Design review of the part built by this model. Coordinates are the model's own, in mm. A direction names the side the tool comes from. Round coordinates to 2 decimals unless told otherwise and drop trailing zeros. Loops run counter-clockwise (first coordinate to the right, second up) from the corner with the lowest first, then second, coordinate; pieces in that order, holes last. Notation, with made-up numbers: (-23, 33.5) - (-17, 33.5) arc R5 ccw to (-17, 41.5) - close; hole circle Ø6 at (28.5, 3). An arc over 180 degrees is marked (long way). Return JSON: item names as keys, results as strings. Group by question number.
(1) Wall thickness on L1, parallel to Z at x = 40, y = 46.75; L2, parallel to Y at x = -31, z = 3; L3, parallel to X at y = 126, z = 0.25: over which ranges is each line inside the solid? List them lowest first. Write a range as [from, to].
(2) We need section D-D, the plane x = 62.5. Write out the cut boundary in (y, z).
(3) We need section B-B, the plane x = -3. Write out the cut boundary in (y, z).
(4) Clearance check with flat-ended pins moving along their axes: pin 1 (4 mm diameter, centred on y = 27, z = -1.5, fed in from +X); pin 2 (6 mm diameter, centred on y = 47.5, z = 2, fed in from +X); pin 3 (10 mm diameter, centred on x = -44.5, y = 31.5, fed in from -Z); pin 4 (2.5 mm diameter, centred on y = 150.5, z = 0, fed in from +X). State where each tip first meets the part, or that it passes through.
(5) We need section C-C, the plane x = -27.5. Write out the cut boundary in (y, z).
(6) The part is to be moulded in two halves that separate along Y. For faces 1 (the flat face through (50, 20, 0)), 2 (the cylindrical face through (73.513, 30.085, 0.056)), 3 (the cylindrical face through (81.638, 112.718, -0.056)), say which applies: pulls with the +Y half, pulls with the -Y half, needs draft (parallel to the pull), parting line crosses it, or undercut.
(7) We need section A-A, the plane y = 85.5. Write out the cut boundary in (x, z), and give its area (3 significant figures).
(8) For faces 4 (the flat face through (1, 40, 0)), 5 (the cylindrical face through (65.185, 14.682, 0.596)), 6 (the flat face through (67.5, 10, 0)), 7 (the cylindrical face through (-0.66, 134.83, -0.06)), list the 3-axis set-ups (+Z, -Z, +X, -X, +Y, -Y) from which the entire face can be reached by the end or side of a thin tool; tool diameter is ignored.
Autodesk Inventor part; units mm, degrees
ref_plane "YZ Plane" through (0, 0, 0) normal (1, 0, 0) x (0, 1, 0)
ref_plane "XZ Plane" through (0, 0, 0) normal (0, 1, 0) x (-1, 0, 0)
ref_plane "XY Plane" through (0, 0, 0) normal (0, 0, 1) x (1, 0, 0)
sketch "Sketch2" plane through (0, 0, 0) normal (0, 0, 1) x (1, 0, 0)
  line L0 (-50, 0) -> (50, 0) construction
  line L1 (50, 0) -> (50, 40)
  line L2 (50, 40) -> (-50, 40)
  line L3 (-50, 40) -> (-50, 0)
  arc A0 (50, 0) -> (-50, 0) centre (0, 74.8331) ccw
  line L4 (57.5, 19.2117) -> (57.5, 34.9113)
  line L5 (-57.5, 34.9113) -> (-57.5, 19.2117)
  line L6 (7.5, 154.4808) -> (7.5, 144.4302)
  line L7 (-7.5, 154.4808) -> (-7.5, 144.4302)
  line L8 (7.5, 144.4302) -> (-7.5, 154.4808) construction
  arc A1 (57.5, 34.9113) -> (7.5, 144.4302) centre (0, 74.8331) ccw
  arc A2 (-7.5, 144.4302) -> (-57.5, 34.9113) centre (0, 74.8331) ccw
  arc A3 (57.5, 19.2117) -> (7.5, 154.4808) centre (0, 74.8331) ccw
  arc A4 (-7.5, 154.4808) -> (-57.5, 19.2117) centre (0, 74.8331) ccw
  line L9 (56.6273, 55) -> (45.8982, 55)
  line L10 (-45.8982, 55) -> (-56.6273, 55)
  line L11 (42.4264, 117.2596) -> (35.3553, 110.1885)
  line L12 (-35.3553, 110.1885) -> (-42.4264, 117.2596)
  line L13 (49.1491, 109.2477) -> (40.9576, 103.512)
  line L14 (-49.1491, 109.2477) -> (-40.9576, 103.512)
  arc A5 (-40.9576, 103.512) -> (-45.8982, 55) centre (0, 74.8331) ccw
  arc A6 (-49.1491, 109.2477) -> (-56.6273, 55) centre (0, 74.8331) ccw
  arc A7 (45.8982, 55) -> (40.9576, 103.512) centre (0, 74.8331) ccw
  arc A8 (35.3553, 110.1885) -> (-35.3553, 110.1885) centre (0, 74.8331) ccw
  arc A9 (56.6273, 55) -> (49.1491, 109.2477) centre (0, 74.8331) ccw
  arc A10 (42.4264, 117.2596) -> (-42.4264, 117.2596) centre (0, 74.8331) ccw
  line L15 (7.5, 114.1237) -> (7.5, 103.8805)
  line L16 (-7.5, 103.8805) -> (-7.5, 114.1237)
  line L17 (34.7368, 55) -> (22.5088, 55)
  line L18 (-22.5088, 55) -> (-34.7368, 55)
  arc A11 (-7.5, 103.8805) -> (-22.5088, 55) centre (0, 74.8331) ccw
  arc A12 (22.5088, 55) -> (7.5, 103.8805) centre (0, 74.8331) ccw
  arc A13 (-7.5, 114.1237) -> (-34.7368, 55) centre (0, 74.8331) ccw
  arc A14 (34.7368, 55) -> (7.5, 114.1237) centre (0, 74.8331) ccw
  point P0 (0, 0)
  point P1 (0, 0)
  point P2 (0, 149.4555)
  dimension "d11" = 100
  dimension "d12" = 40
  dimension "d27" = 90
  dimension "d29" = 7.5
  dimension "d30" = 7.5
  dimension "d34" = 10
  dimension "d35" = 10
  dimension "d36" = 10
  dimension "d37" = 10
  dimension "d38" = 15
  dimension "d71" = 15
  dimension "d74" = 10
  dimension "d75" = 10
  dimension "d76" = 45
  dimension "d77" = 45
  dimension "d78" = 10
  dimension "d79" = 10
  dimension "d80" = 10
  dimension "d81" = 10
extrude "Extrusion2" add sketch "Sketch2" along normal mid plane 8
sketch "Sketch6" plane through (0, 0, 0) normal (0, 0, 1) x (1, 0, 0)
  arc A0 (50, 0) -> (-50, 0) centre (0, 74.8331) ccw
  line L0 (57.5, 5.5962) -> (67.5, 5.5962)
  line L1 (67.5, 5.5962) -> (67.5, 15.3037)
  point P0 (0, 0)
  point P1 (57.5, 19.2117)
  dimension "d48" = 10
extrude "Extrusion4" add sketch "Sketch6" along normal mid plane 10
sketch "Sketch8" plane through (0, 0, 0) normal (0, 0, 1) x (1, 0, 0)
  arc A0 (50, 0) -> (-50, 0) centre (0, 74.8331) ccw construction
  line L0 (2, 165.8331) -> (0, 163.8331)
  line L1 (0, 163.8331) -> (-2, 165.8331)
  line L2 (-2, 165.8331) -> (2, 165.8331)
  line L3 (0, 165.8331) -> (0, 164.8331) construction
  point P0 (0, 0)
  point P1 (67.5, 15.3037)
  dimension "d67" = 1
  dimension "d68" = 2
extrude "Extrusion5" cut sketch "Sketch8" along normal mid plane 10
sketch "Sketch7" plane through (57.5, 5.5962, 5) normal (0, -1, 0) x (1, 0, 0)
  line L0 (10, 0) -> (10, -10)
  line L1 (0, 0) -> (10, 0)
  line L2 (10, -10) -> (0, -10)
  line L3 (0, 0) -> (10, -10)
  line L4 (0, -9) -> (0, -1)
  line L5 (0, -1) -> (0, 0)
  line L6 (0, -10) -> (0, -9)
  point P0 (-57.5, -5)
  point P1 (5, -5)
hole "Hole2" at (62.5, 5.5962, 0) direction (0, 1, 0) diameter 5.5 depth 25 tip angle 118
sketch "Sketch9" plane through (0, 0, -4) normal (0, 0, -1) x (-1, 0, 0)
  arc A0 (-0.9945, 164.8277) -> (-67.5, 15.3037) centre (0, 74.8331) ccw construction
  line L0 (-73.6122, 32.3331) -> (0, 74.8331) construction
  line L1 (0, 74.8331) -> (0, 98.0248) construction
  point P0 (0, 0)
  dimension "d82" = 85
  dimension "d83" = 120
hole "Hole3" at (73.6122, 32.3331, -4) direction (0, 0, 1) diameter 4.5 depth 10 tip angle 118
pattern_circular "Circular Pattern2" count 6 over 110 about axis through (0, 74.8331, 0) along (0, 0, 1) of "Hole3"
sketch "Sketch10" plane through (-50, 40, 4) normal (0, -1, 0) x (1, 0, 0)
  line L0 (90, -4.6611) -> (50, -4) construction
  line L1 (50, -4) -> (10, -3.3389) construction
  dimension "d94" = 80
hole "Hole4" at (-40, 40, 0.6611) at (40, 40, -0.6611) direction (0, 1, 0) diameter 3.242 depth 11.8 tip angle 118
sketch "Sketch11" plane through (0, 0, -4) normal (0, 0, -1) x (-1, 0, 0)
  point P0 (0, 0)
sketch "Sketch12" plane through (0, 0, -4) normal (0, 0, -1) x (-1, 0, 0)
  arc A0 (22.5088, 55) -> (7.5, 103.8805) centre (0, 74.8331) ccw construction
  line L0 (0, 74.8331) -> (12.608, 74.8331) construction
  point P0 (0, 0)
  point P1 (14.7601, 158.5418)
  point P2 (60.1041, 14.7291)
  point P3 (49.7929, 116.6143)
  point P4 (8, 49.8331)
  dimension "d102" = 85
  dimension "d103" = 65
  dimension "d104" = 85
  dimension "d105" = 80
  dimension "d106" = 40
  dimension "d107" = 45
  dimension "d108" = 25
  dimension "d109" = 8
hole "Hole5" at (-14.7601, 158.5418, -4) at (-49.7929, 116.6143, -4) at (-8, 49.8331, -4) at (-60.1041, 14.7291, -4) direction (0, 0, 1) diameter 3.5 depth 11.8 tip angle 118
equation "\"d36\" = d35"
equation "\"d37\" = d34"
properties part number "M02_R01 - Main Spherical Shaft" material "Glass"
Solutions:
{
 "1": {"L1": "[-4, -2.28], [0.96, 4]", "L2": "[40, 55], [100.11, 114.06], [126.2, 137.59], [148.58, 159.33]", "L3": "[-74.04, -61.5], [-47.77, -31.34], [31.34, 47.77], [61.5, 66.87], [70.67, 74.04]"},
 "2": {"outline": "(5.6, -5) - (10.07, -5) - (10.07, -4) - (24.9, -4) - (24.9, -2.75) - (5.6, -2.75) - close; (5.6, 2.75) - (24.9, 2.75) - (24.9, 4) - (10.07, 4) - (10.07, 5) - (5.6, 5) - close; (43.31, -4) - (106.36, -4) - (106.36, 4) - (43.31, 4) - close; (124.77, -4) - (139.59, -4) - (139.59, 4) - (124.77, 4) - close"},
 "3": {"outline": "(40, -4) - (124.74, -4) - (124.74, 4) - (40, 4) - close; (134.76, -4) - (164.78, -4) - (164.78, 4) - (134.76, 4) - close"},
 "4": {"pin 1": "x = 77.46", "pin 2": "x = 86.65", "pin 3": "through", "pin 4": "x = 50.62"},
 "5": {"outline": "(40, -4) - (55, -4) - (55, 4) - (40, 4) - close; (62.84, -4) - (86.82, -4) - (86.82, 4) - (62.84, 4) - close; (103.88, -4) - (116.59, -4) - (116.59, 4) - (103.88, 4) - close; (128.16, -4) - (139.21, -4) - (139.21, 4) - (128.16, 4) - close; (149.96, -4) - (160.53, -4) - (160.53, 4) - (149.96, 4) - close"},
 "6": {"face 1": "needs draft", "face 2": "undercut", "face 3": "parting line crosses it"},
 "7": {"outline": "(-89.37, -4) - (-79.29, -4) - (-79.29, 4) - (-89.37, 4) - close; (-69.18, -4) - (-59.04, -4) - (-59.04, 4) - (-69.18, 4) - close; (-48.85, -4) - (-38.55, -4) - (-38.55, 4) - (-48.85, 4) - close; (-28.04, -4) - (28.04, -4) - (28.04, 4) - (-28.04, 4) - close; (38.55, -4) - (48.85, -4) - (48.85, 4) - (38.55, 4) - close; (59.04, -4) - (69.18, -4) - (69.18, 4) - (59.04, 4) - close; (79.29, -4) - (89.37, -4) - (89.37, 4) - (79.29, 4) - close", "area": "937 mm^2"},
 "8": {"face 4": "+Z, -Z, -Y", "face 5": "-Y", "face 6": "+Z, -Z, +X, -Y", "face 7": "+Z, -Z"}
}
